from build123d import *

# Parameters (mm, degrees)
F0_R     = 1.75
F0_R_2   = 4.5
F1_DEPTH = 2
F2_R     = 3


with BuildPart() as f1:
    # F0 (on Top) → F1 (new body)
    with BuildSketch(Plane.XY):
        with BuildLine():
            Line((20, 30), (-20, 30))
            Line((-20, 30), (-20, 22))
            ThreePointArc((-20, 22), (-13.8300253787, 0), (-20, -22))
            Line((-20, -22), (-20, -30))
            Line((-20, -30), (20, -30))
            Line((20, -30), (20, -22))
            ThreePointArc((20, -22), (13.8300253787, 0), (20, 22))
            Line((20, 22), (20, 30))
        make_face()
        with Locations((-16, -26)):
            Circle(F0_R, mode=Mode.SUBTRACT)
        with Locations((-6.4855394704, -3.7666666667)):
            Circle(F0_R, mode=Mode.SUBTRACT)
        Polygon((10, -22.4003139883), (0, -22.4003139883), (-10, -22.4003139883), (0, -11.7255505174), align=None, mode=Mode.SUBTRACT)
        with Locations((16, -26)):
            Circle(F0_R, mode=Mode.SUBTRACT)
        with Locations((6.4855394704, -3.7666666667)):
            Circle(F0_R, mode=Mode.SUBTRACT)
        with Locations((-16, 26)):
            Circle(F0_R, mode=Mode.SUBTRACT)
        Circle(F0_R_2, mode=Mode.SUBTRACT)
        with Locations((0, 7.5)):
            Circle(F0_R, mode=Mode.SUBTRACT)
        Polygon((0, 22.4003139883), (10, 22.4003139883), (0, 11.7255505174), (-10, 22.4003139883), align=None, mode=Mode.SUBTRACT)
        with Locations((16, 26)):
            Circle(F0_R, mode=Mode.SUBTRACT)
    extrude(amount=F1_DEPTH)

    # F2
    f2_edges = [f1.edges().sort_by_distance(p)[0] for p in [
        (-20, 30, 1),
        (-20, -30, 1),
        (20, -30, 1),
        (20, 30, 1),
        (20, -22, 1),
        (-20, -22, 1),
        (-20, 22, 1),
    ]]
    fillet(f2_edges, radius=F2_R)


solid = f1.part
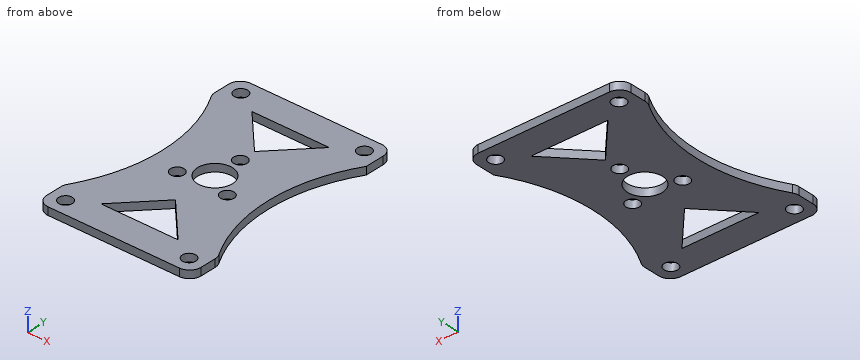
The listing builds one solid part. Answer for the finished solid, in the listing's coordinates (mm). Round coordinates to 2 decimals unless told otherwise and drop trailing zeros. Loops run counter-clockwise (first coordinate to the right, second up) from the corner with the lowest first, then second, coordinate; pieces in that order, holes last. Notation, with made-up numbers: M -7.5,45.5 L 29.5,45.5 A13 ccw 29.5,57.5 Z; hole C 47,75.5 d8. An arc over 180 degrees is marked long. Write each question's results on one line, items separated by ' | '. Start each with the question number.
1) Find section D-D on z = 0.3. Count the separate pieces of the cut face and the enclosed holes in it, plus the area to 3 significant figures.
2) This flat-tipped pin is pushed along its axis until it touches: pin 1 (3 mm diameter, centred on x = -16, y = -26, fed in from +Z). Where does it stop, or does it pass through?
3) Find section A-A on y = -26. Write down the section's boundary in (x, z).
4) Straight lines are drawn through the part: probe 1 along Y at (x, z) = (3, 1.25); probe 2 along Y at (x, z) = (5, 0.3); probe 3 along X at (y, z) = (-17, 1). For each, find the intervals that lie inside material, in ascending order.
5) Find section B-B on y = 0. Write down the section's boundary in (x, z), plus the area to 3 significant figures.
6) Find section C-C on x = 16. Write down the section's boundary in (y, z), plus the area to 3 significant figures.
Final values:
1) separate pieces: 1 | enclosed holes: 10 | area: 1,680 mm²
2) pin 1: through
3) outline: M -20,0 L -17.75,0 L -17.75,2 L -20,2 Z; M -14.25,0 L 14.25,0 L 14.25,2 L -14.25,2 Z; M 17.75,0 L 20,0 L 20,2 L 17.75,2 Z
4) probe 1: -30 to -22.4, -14.93 to -3.35, 3.35 to 14.93, 22.4 to 30 | probe 2: -30 to -22.4, -17.06 to -4.69, -2.84 to 17.06, 22.4 to 30 | probe 3: -17.4 to -4.94, 4.94 to 17.4
5) outline: M -13.83,0 L -4.5,0 L -4.5,2 L -13.83,2 Z; M 4.5,0 L 13.83,0 L 13.83,2 L 4.5,2 Z | area: 37.3 mm²
6) outline: M -30,0 L -27.75,0 L -27.75,2 L -30,2 Z; M -24.25,0 L -13.38,0 L -13.38,2 L -24.25,2 Z; M 13.38,0 L 24.25,0 L 24.25,2 L 13.38,2 Z; M 27.75,0 L 30,0 L 30,2 L 27.75,2 Z | area: 52.5 mm²
